Geometry check sheet. Reference: drawing and pictorial views, mm from the part's lowest x, y, z. Give positions to 0.01 mm unless a question says otherwise; leave off trailing zeros. Order: outer loops, then holes, each group sorted by start corner. A loop starts at its lowest first (then second) coordinate and runs counter-clockwise, first axis right, second up.
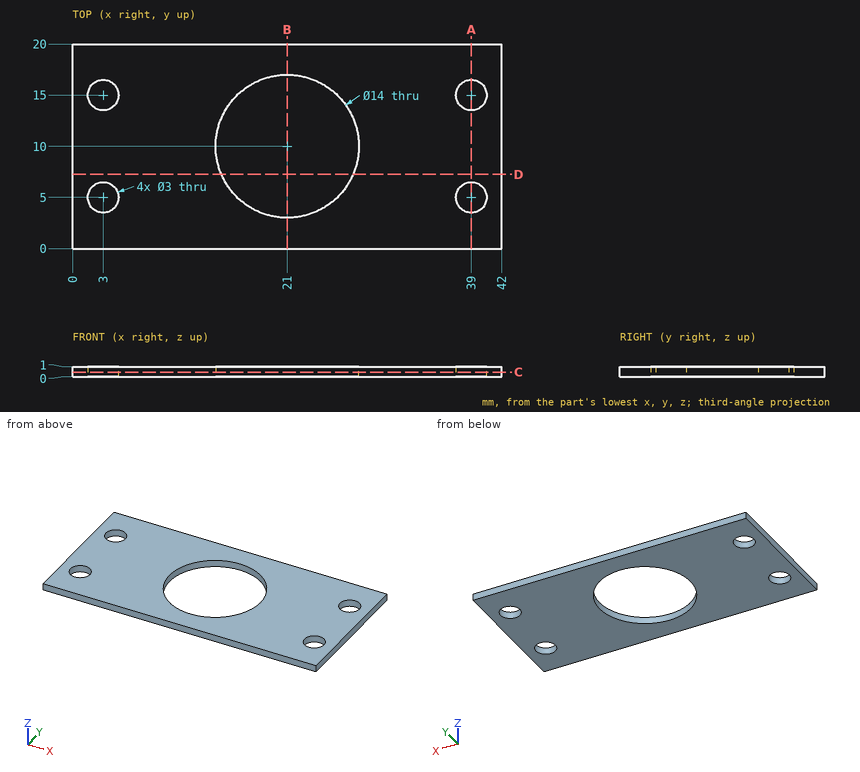
1) Section check A-A, the plane x = 39. Record the cut outline in (y, z), then the cut area to 3 significant figures.
Recorded:
outline: (0, 0) - (3.5, 0) - (3.5, 1) - (0, 1) - close; (6.5, 0) - (13.5, 0) - (13.5, 1) - (6.5, 1) - close; (16.5, 0) - (20, 0) - (20, 1) - (16.5, 1) - close
area: 14.0 mm2
2) Material ranges on L1, parallel to Y at x = 3, z = 0.6; L2, parallel to X at y = 5, z = 0.35; L3, parallel to Y at x = 21, z = 0.7, recorded low to high.
Recorded:
L1: y = 0 to 3.5, 6.5 to 13.5, 16.5 to 20
L2: x = 0 to 1.5, 4.5 to 16.1, 25.9 to 37.5, 40.5 to 42
L3: y = 0 to 3, 17 to 20
3) Section check D-D, the plane y = 7.25. Record the cut outline in (x, z).
Recorded:
outline: (0, 0) - (14.56, 0) - (14.56, 1) - (0, 1) - close; (27.44, 0) - (42, 0) - (42, 1) - (27.44, 1) - close
4) Section check B-B, the plane x = 21. Record the cut outline in (y, z), then the cut area to 3 significant figures.
Recorded:
outline: (0, 0) - (3, 0) - (3, 1) - (0, 1) - close; (17, 0) - (20, 0) - (20, 1) - (17, 1) - close
area: 6.00 mm2
5) Section check C-C, the plane z = 0.45. Record the cut outline in (x, y).
Recorded:
outline: (0, 0) - (42, 0) - (42, 20) - (0, 20) - close; hole circle Ø3 at (3, 5); hole circle Ø3 at (3, 15); hole circle Ø14 at (21, 10); hole circle Ø3 at (39, 5); hole circle Ø3 at (39, 15)
